from build123d import *

# Parameters (mm, degrees)
AUFSATZ_LINEAR_AUSTRAGEN1_DEPTH = 5
SKIZZE2_R                       = 50
SCHNITT_LINEAR_AUSTRAGEN1_DEPTH = 384.666521865
AUFSATZ_LINEAR_START            = 15
AUFSATZ_LINEAR_AUSTRAGEN2_DEPTH = 15
SKIZZE4_R                       = 3.6
SCHNITT_LINEAR_AUSTRAGEN2_DEPTH = 4.4
SCHNITT_LINEAR_AUSTRAGEN3_DEPTH = 384.927076409


with BuildPart() as part:
    # Skizze1 → Aufsatz-Linear austragen1 (new body)
    with BuildSketch(Plane(origin=(0, 0, 0), x_dir=(1, 0, 0), z_dir=(0, 1, 0))):
        with BuildLine():
            Line((150, 0), (290, 0))
            ThreePointArc((290, 0), (251.147367097, 145), (145, 251.147367097))
            Line((145, 251.147367097), (75, 129.903810568))
            ThreePointArc((75, 129.903810568), (129.903810568, 75), (150, 0))
        make_face()
    extrude(amount=AUFSATZ_LINEAR_AUSTRAGEN1_DEPTH)

    # Skizze2 → Schnitt-Linear austragen1 (cut, through all)
    with BuildSketch(Plane(origin=(0, 5, 0), x_dir=(1, 0, 0), z_dir=(0, 1, 0))):
        with Locations(Location((217.333310915, 58.234285148, 0), (0, 0, 270))):
            Circle(SKIZZE2_R)
        with Locations(Location((159.099025767, 159.099025767, 0), (0, 0, 270))):
            Circle(SKIZZE2_R)
    extrude(amount=-SCHNITT_LINEAR_AUSTRAGEN1_DEPTH, mode=Mode.SUBTRACT)

    # Skizze3 → Aufsatz-Linear austragen2 (add)
    with BuildSketch(Plane(origin=(0, 5, 0), x_dir=(1, 0, 0), z_dir=(0, 1, 0)).offset(AUFSATZ_LINEAR_START)):
        with BuildLine():
            Line((146.158073512, 110.802734453), (144.863978286, 105.973105321))
            ThreePointArc((144.863978286, 105.973105321), (194.4523443, 116.966581395), (213.889734162, 163.892591618))
            Line((213.889734162, 163.892591618), (208.908760672, 163.456812904))
            ThreePointArc((208.908760672, 163.456812904), (191.238406251, 120.796803611), (146.158073512, 110.802734453))
        make_face()
        with BuildLine():
            Line((181.977971856, 22.878946089), (178.44243795, 19.343412183))
            ThreePointArc((178.44243795, 19.343412183), (226.883960687, 4.069858732), (267.180239202, 34.990280752))
            Line((267.180239202, 34.990280752), (262.648700267, 37.103372061))
            ThreePointArc((262.648700267, 37.103372061), (226.015719798, 8.993897497), (181.977971856, 22.878946089))
        make_face()
    extrude(amount=-AUFSATZ_LINEAR_AUSTRAGEN2_DEPTH)

    # Skizze4 → Schnitt-Linear austragen2 (cut)
    with BuildSketch(Plane.XZ):
        with Locations(Location((277.604561185, -36.547333822, 0), (0, 0, 270))):
            Circle(SKIZZE4_R)
        with Locations(Location((258.686269103, -107.151361062, 0), (0, 0, 270))):
            Circle(SKIZZE4_R)
        with Locations(Location((222.138935282, -170.453200122, 0), (0, 0, 270))):
            Circle(SKIZZE4_R)
        with Locations(Location((170.453200122, -222.138935282, 0), (0, 0, 270))):
            Circle(SKIZZE4_R)
        with Locations(Location((103.489442931, -134.87006785, 0), (0, 0, 270))):
            Circle(SKIZZE4_R)
        with Locations(Location((134.87006785, -103.489442931, 0), (0, 0, 270))):
            Circle(SKIZZE4_R)
        with Locations(Location((168.545626434, -22.189452677, 0), (0, 0, 270))):
            Circle(SKIZZE4_R)
        with Locations(Location((157.059520527, -65.056183502, 0), (0, 0, 270))):
            Circle(SKIZZE4_R)
    extrude(amount=-SCHNITT_LINEAR_AUSTRAGEN2_DEPTH, mode=Mode.SUBTRACT)

    # Skizze5 → Schnitt-Linear austragen3 (cut, through all)
    with BuildSketch(Plane(origin=(0, 5, 0), x_dir=(1, 0, 0), z_dir=(0, 1, 0))):
        with BuildLine():
            Line((75, 129.903810568), (82.5, 142.894191624))
            Line((82.5, 142.894191624), (88.995190528, 139.144191624))
            Line((88.995190528, 139.144191624), (81.401381861, 125.99132919))
            ThreePointArc((81.401381861, 125.99132919), (78.225155415, 127.987597291), (75, 129.903810568))
        make_face()
        with BuildLine():
            Line((150, 0), (165, 0))
            Line((165, 0), (165, 7.5))
            Line((165, 7.5), (149.812382666, 7.5))
            ThreePointArc((149.812382666, 7.5), (149.953088331, 3.751173159), (150, 0))
        make_face()
        with BuildLine():
            Line((125.99132919, 81.401381861), (139.144191624, 88.995190528))
            Line((139.144191624, 88.995190528), (146.644191624, 76.004809472))
            Line((146.644191624, 76.004809472), (133.49132919, 68.411000805))
            ThreePointArc((133.49132919, 68.411000805), (129.903810568, 75), (125.99132919, 81.401381861))
        make_face()
    extrude(amount=-SCHNITT_LINEAR_AUSTRAGEN3_DEPTH, mode=Mode.SUBTRACT)


solid = part.part
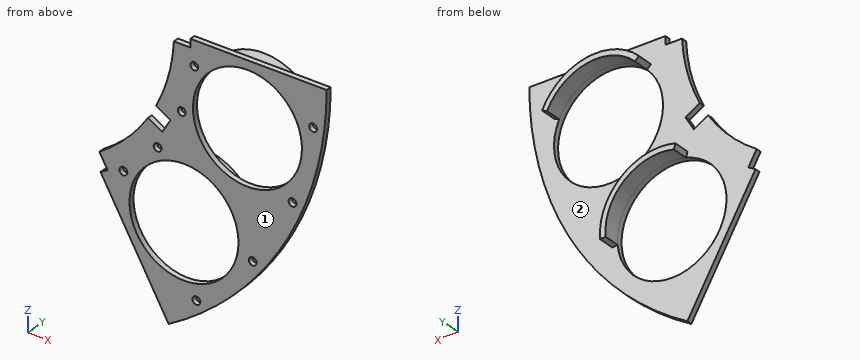
The model under review builds one solid part; all positions refer to its coordinate system, in mm. Face numbers are marked on the shaded views. A direction names the side the tool comes from. Coordinates: 2 decimals unless noted, no trailing zeros. Write each loop counter-clockwise with the first axis right and the second up, starting at its lowest first coordinate (ties: lowest second). Pieces come first, ordered by that corner, then holes. Notation, with made-up numbers: (15.5, -32.75) - (36.5, -32.75) arc R20 cw to (36.5, -2.75) - close; hole circle Ø9 at (20, -18.5). An arc over 180 degrees is marked (long way). Answer as a JSON object with one key per item and string values. Group by question number.
1. Add section A-A (y = 8.25). Give the boundary of the cut face in (x, z).
2. Add section C-C (x = 205). Give the boundary of the cut face in (y, z).
3. Add section D-D (x = 118.5). Give the boundary of the cut face in (y, z).
4. Add section B-B (z = -120.5). Give the boundary of the cut face in (x, y), plus the area to 3 significant figures.
5. Machinability: for the marked faces 1 and 2, which of the approach directions +Z, -Z, +X, -X, +Y, -Y give a long, thin tool a straight path to every point of the face, cutting with its end or side? Answer none if there is none.
6. To check wall thickness, follow probe 1 along Z at (x, y) = (160, 4); probe 2 along Z at (x, y) = (136, 2); probe 3 along Y at (x, z) = (157, -12). State the ranges of each line that lie inside material, in increasing order.
7. Clearance check with flat-ended pins moving along their axes: pin 1 Ø6.5 at (x, z) = (168.55, -22.19) entering from +Y; pin 2 Ø1 at (x, y) = (171.5, 12) entering from +Z; pin 3 Ø2 at (y, z) = (7, -128) entering from +X. State where each tip first meets the part, or that it passes through.
Findings:
{
 "1": {"outline": "(144.86, -105.97) - (146.16, -110.8) arc R50 cw to (208.91, -163.46) - (213.89, -163.89) arc R55 ccw to start; (178.44, -19.34) - (181.98, -22.88) arc R50 cw to (262.65, -37.1) - (267.18, -34.99) arc R55 ccw to start"},
 "2": {"outline": "(0, -205.12) - (5, -205.12) - (5, -178.93) - (0, -178.93) - close; (0, -139.27) - (20, -139.27) - (20, -128.8) - (5, -128.8) - (5, -106.69) - (0, -106.69) - close; (0, -9.78) - (20, -9.78) - (20, -4.63) - (5, -4.63) - (5, 0) - (0, 0) - close"},
 "3": {"outline": "(0, -205.25) - (5, -205.25) - (5, -188.28) - (0, -188.28) - close; (0, -129.91) - (5, -129.91) - (5, -91.97) - (0, -91.97) - close"},
 "4": {"outline": "(89.33, 0) - (127.32, 0) - (127.32, 5) - (89.33, 5) - close; (190.88, 0) - (263.78, 0) - (263.78, 5) - (198.28, 5) - (198.28, 20) - (190.88, 20) - close", "area": "665 mm²"},
 "5": {"face 1": "+Z, -Z, +X, -X, -Y", "face 2": "+Y"},
 "6": {"probe 1": "-241.87 to -209.09, -109.11 to -67.13, -62.98 to -7.5", "probe 2": "-235.56 to -203.44, -114.75 to -106.91, -100.07 to -87.18, -69.86 to -63.28", "probe 3": "0 to 5"},
 "7": {"pin 1": "y = 5", "pin 2": "z = -105.4", "pin 3": "x = 205.13"}
}
